Could you check a few things on this model? Use its own coordinates, in mm. A direction names the side the tool comes from. Round coordinates to 2 decimals unless told otherwise and drop trailing zeros. Order: outer loops, then holes, each group sorted by start corner. A loop starts at its lowest first (then second) coordinate and runs counter-clockwise, first axis right, second up.
```python
from build123d import *

# Parameters (mm, degrees)
BOSS_EXTRUDE1_DEPTH = 12.7
SKETCH2_W           = 12.7
SKETCH2_H           = 6.35
BOSS_EXTRUDE2_DEPTH = 101.6
BOSS_EXTRUDE3_REACH = 105.182
SKETCH3_R           = 19.05


with BuildPart() as part:
    # Sketch1 → Boss-Extrude1 (new body)
    with BuildSketch(Plane(origin=(0, 0, 0), x_dir=(1, 0, 0), z_dir=(0, 1, 0))):
        with BuildLine():
            Line((0, 50.8), (76.2, 50.8))
            Line((76.2, 50.8), (76.2, -50.8))
            Line((76.2, -50.8), (0, -50.8))
            ThreePointArc((0, -50.8), (-50.8, 0), (0, 50.8))
        make_face()
    extrude(amount=BOSS_EXTRUDE1_DEPTH)

    # Sketch2 → Boss-Extrude2 (add)
    with BuildSketch(Plane.XY.offset(50.8)):
        with Locations((69.85, -3.175)):
            Rectangle(SKETCH2_W, SKETCH2_H)
    extrude(amount=-BOSS_EXTRUDE2_DEPTH)

    # Boss-Extrude3: up to this face of the body (flat: up to its plane)
    boss_extrude3_end = Plane(part.part.faces().sort_by_distance((17.597225425, 12.7, 0))[0])
    # Sketch3 → Boss-Extrude3 (add, up to the picked face)
    with BuildSketch(Plane(origin=(24.549261314, 42.520567884, 0), x_dir=(0, 0, -1), z_dir=(0.500000000000001, 0.866025403784438, 0)), mode=Mode.PRIVATE) as boss_extrude3_sk1:
        with BuildLine():
            Line((-38.1, 3.858864232), (-38.1, -59.641135768))
            Line((-38.1, -59.641135768), (38.1, -59.641135768))
            Line((38.1, -59.641135768), (38.1, 3.858864232))
            ThreePointArc((38.1, 3.858864232), (0, 41.958864232), (-38.1, 3.858864232))
        make_face()
        with Locations(Location((0, 3.858864232, 0), (0, 0, 90))):
            Circle(SKETCH3_R, mode=Mode.SUBTRACT)
    boss_extrude3_tool1 = split(extrude(boss_extrude3_sk1.sketch, amount=-BOSS_EXTRUDE3_REACH, mode=Mode.PRIVATE), bisect_by=boss_extrude3_end, keep=Keep.BOTH, mode=Mode.PRIVATE)
    add(boss_extrude3_tool1.solids().sort_by(Axis((38.119708, 34.685667, 0), (-0.500000000000001, -0.866025403784438, 0)))[0])


solid = part.part
```
Q1. Imagine slicing it at C-C, the plane y = 11. Please give me the cut outline in (x, z), then the cut area to 3 significant figures.
Q2. Imagine slicing it at B-B, the plane x = 56.5. Please give me the cut outline in (y, z), then the cut area to 3 significant figures.
Q3. Imagine slicing it at A-A, the plane z = -9. Please give me the cut outline in (x, y), then the cut area to 3 significant figures.
Q4. I need wall thicknesses on L1, parallel to Y at x = -26, z = 38.5; L2, parallel to X at y = 13.5, z = -13; L3, parallel to X at y = 17, z = 7. Which ranges of each line are inside material? Lowest first, please.
Q5. We'd pull the mould along Y, two halves only. Please class faces 1 (the cylindrical face through (-3.63, 37.77, 5.72)), 2 (the cylindrical face through (-50.788, 6.261, 1.117)), 3 (the flat face through (70, -6.35, 1)): released by +Y, released by -Y, zero draft, split by the parting line, or undercut.
Q6. Imagine slicing it at D-D, the plane z = -25. Please give me the cut outline in (x, y).
Q7. For P1, Ø1.9, axis at y = -3, z = -23.5, coming from the -X side; P2, Ø11.5, axis at x = 13.5, z = -0.5, coming from the +Y side; P3, Ø9.5, axis at x = 22.5, y = 21.5, coming from the -Z side, each with a flat end and sliding along its axis, tell me the tip position at first contact or that it passes through.
Q8. For faces 4 (the flat face through (-6, 12.7, -38)), 5 (the flat face through (35, 20, 38.1)), 6 (the flat face through (32, 27, -38.1)), 7 (the flat face through (63.5, -3, 1)), which set-ups out of +Z, -Z, +X, -X, +Y, -Y let a thin tool reach every point of the face, with its end or its side?
Filled in:
1. outline: (0, -50.8) - (76.2, -50.8) - (76.2, 50.8) - (0, 50.8) arc R50.8 ccw to start
1. area: 11,800 mm2
2. outline: (0, -50.8) - (12.7, -50.8) - (12.7, -38.1) - (24.07, -38.1) - (24.07, 38.1) - (12.7, 38.1) - (12.7, 50.8) - (0, 50.8) - close
2. area: 2,160 mm2
3. outline: (-50, 0) - (63.5, 0) - (63.5, -6.35) - (76.2, -6.35) - (76.2, 12.7) - (35.75, 36.06) - (22.26, 12.7) - (-16.51, 12.7) - (6.67, 52.84) - (-10.85, 62.96) - (-39.87, 12.7) - (-50, 12.7) - close
3. area: 3,370 mm2
4. L1: y = 0 to 12.7
4. L2: x = -38.02 to -12.74, 19.42 to 74.81
4. L3: x = -37.89 to -15.1, 25.82 to 68.75
5. face 1: undercut
5. face 2: zero draft
5. face 3: released by -Y
6. outline: (-44.22, 0) - (63.5, 0) - (63.5, -6.35) - (76.2, -6.35) - (76.2, 12.7) - (-3.69, 58.83) - (-30.32, 12.7) - (-44.22, 12.7) - close
7. P1: stops at x = 63.5
7. P2: stops at y = 12.7
7. P3: stops at z = -38.1
8. face 4: -X, +Y
8. face 5: +Z, +X, -X, +Y
8. face 6: -Z, +X, -X, +Y
8. face 7: +Z, -Z, -X, -Y
